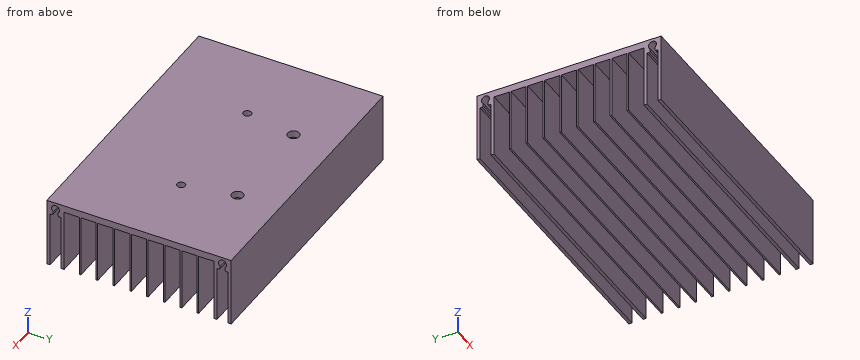
```python
from build123d import *

# Parameters (mm, degrees)
SCHIZZO1_W                   = 120
SCHIZZO1_H                   = 80
ESTRUSIONE_ESTRUSIONE1_DEPTH = 30
SCHIZZO2_W                   = 27
SCHIZZO2_H                   = 6.6
TAGLIO_ESTRUSIONE1_DEPTH     = 121
RIPETIZIONE_A_L1_COUNT       = 9
RIPETIZIONE_A_L1_PITCH       = 7.3
SCHIZZO3_W                   = 24
SCHIZZO3_H                   = 4.7
TAGLIO_ESTRUSIONE2_DEPTH     = 121
TAGLIO_ESTRUSIONE3_DEPTH     = 121
SMUSSO1_SIZE                 = 0.5
SCHIZZO5_R                   = 1.75
SCHIZZO5_R_2                 = 2.5
TAGLIO_ESTRUSIONE4_DEPTH     = 10


with BuildPart() as part:
    # Schizzo1 → Estrusione-Estrusione1 (new body)
    with BuildSketch(Plane.XY):
        Rectangle(SCHIZZO1_W, SCHIZZO1_H)
    extrude(amount=ESTRUSIONE_ESTRUSIONE1_DEPTH)

    # Schizzo2 → Taglio-Estrusione1 (cut, through all)
    with BuildSketch(Plane.ZY.offset(60)):
        with Locations((13.5, -29.2)):
            Rectangle(SCHIZZO2_W, SCHIZZO2_H)
    taglio_estrusione1 = extrude(amount=-TAGLIO_ESTRUSIONE1_DEPTH, mode=Mode.SUBTRACT)

    # Ripetizione a L1: Taglio-Estrusione1 ×9
    with Locations(*[(0, i * RIPETIZIONE_A_L1_PITCH, 0) for i in range(1, RIPETIZIONE_A_L1_COUNT)]):
        add(taglio_estrusione1, mode=Mode.SUBTRACT)

    # Schizzo3 → Taglio-Estrusione2 (cut, through all)
    with BuildSketch(Plane(origin=(60, 0, 0), x_dir=(0, 0, -1), z_dir=(1, 0, 0))):
        with Locations((-12, -36.25)):
            Rectangle(SCHIZZO3_W, SCHIZZO3_H)
        with Locations((-12, 36.25)):
            Rectangle(SCHIZZO3_W, SCHIZZO3_H)
    extrude(amount=-TAGLIO_ESTRUSIONE2_DEPTH, mode=Mode.SUBTRACT)

    # Schizzo4 → Taglio-Estrusione3 (cut, through all)
    with BuildSketch(Plane(origin=(60, 0, 0), x_dir=(0, 0, -1), z_dir=(1, 0, 0))):
        with BuildLine():
            ThreePointArc((-25.3, 36.25), (-25.38030749, 35.725951413), (-25.613859338, 35.25))
            Line((-25.613859338, 35.25), (-24, 35.25))
            Line((-24, 35.25), (-24, 37.25))
            Line((-24, 37.25), (-25.613859338, 37.25))
            ThreePointArc((-25.613859338, 37.25), (-25.38030749, 36.774048587), (-25.3, 36.25))
        make_face()
        with BuildLine():
            Line((-27.05, 37.25), (-27.05, 35.25))
            Line((-27.05, 35.25), (-25.613859338, 35.25))
            ThreePointArc((-25.613859338, 35.25), (-25.38030749, 35.725951413), (-25.3, 36.25))
            ThreePointArc((-25.3, 36.25), (-25.38030749, 36.774048587), (-25.613859338, 37.25))
            Line((-25.613859338, 37.25), (-27.05, 37.25))
        make_face()
        with BuildLine():
            Line((-25.613859338, 35.25), (-27.05, 35.25))
            Line((-27.05, 35.25), (-27.05, 37.25))
            Line((-27.05, 37.25), (-25.613859338, 37.25))
            ThreePointArc((-25.613859338, 37.25), (-28.8, 36.25), (-25.613859338, 35.25))
        make_face()
        with BuildLine():
            ThreePointArc((-25.3, -36.25), (-25.38030749, -35.725951413), (-25.613859338, -35.25))
            Line((-25.613859338, -35.25), (-27.05, -35.25))
            Line((-27.05, -35.25), (-27.05, -37.25))
            Line((-27.05, -37.25), (-25.613859338, -37.25))
            ThreePointArc((-25.613859338, -37.25), (-25.38030749, -36.774048587), (-25.3, -36.25))
        make_face()
        with BuildLine():
            Line((-27.05, -35.25), (-25.613859338, -35.25))
            ThreePointArc((-25.613859338, -35.25), (-28.8, -36.25), (-25.613859338, -37.25))
            Line((-25.613859338, -37.25), (-27.05, -37.25))
            Line((-27.05, -37.25), (-27.05, -35.25))
        make_face()
        with BuildLine():
            Line((-24, -37.25), (-24, -35.25))
            Line((-24, -35.25), (-25.613859338, -35.25))
            ThreePointArc((-25.613859338, -35.25), (-25.38030749, -35.725951413), (-25.3, -36.25))
            ThreePointArc((-25.3, -36.25), (-25.38030749, -36.774048587), (-25.613859338, -37.25))
            Line((-25.613859338, -37.25), (-24, -37.25))
        make_face()
    extrude(amount=-TAGLIO_ESTRUSIONE3_DEPTH, mode=Mode.SUBTRACT)

    # Smusso1
    smusso1_edges = [part.edges().sort_by_distance(p)[0] for p in [
        (0, 37.25, 24),
        (0, 35.25, 24),
        (0, -35.25, 24),
        (0, -37.25, 24),
    ]]
    chamfer(smusso1_edges, length=SMUSSO1_SIZE)

    # Schizzo5 → Taglio-Estrusione4 (cut)
    with BuildSketch(Plane.XY.offset(30)):
        with Locations((-25.5, 0)):
            Circle(SCHIZZO5_R)
        with Locations((26.686198964, 0)):
            Circle(SCHIZZO5_R)
        with Locations((-21.944553743, 22)):
            Circle(SCHIZZO5_R_2)
        with Locations((22.18196976, 22)):
            Circle(SCHIZZO5_R_2)
    extrude(amount=-TAGLIO_ESTRUSIONE4_DEPTH, mode=Mode.SUBTRACT)


solid = part.part
```
Here's how the part is built. I have some questions about the finished solid (model axes, mm). Coordinates: 2 decimals unless noted, no trailing zeros. Order: outer loops, then holes, each group sorted by start corner. A loop starts at its lowest first (then second) coordinate and runs counter-clockwise, first axis right, second up.
1) Imagine slicing it at C-C on y = 22. List the corners of the cut face in (x, z) for me.
2) Imagine slicing it at B-B on z = 11.25. State how many separate pieces and enclosed holes the cut face has, and give its area (3 significant figures).
3) Imagine slicing it at A-A on y = 0. List the corners of the cut face in (x, z) for me.
4) Imagine slicing it at D-D on y = -28. List the corners of the cut face in (x, z) for me.
5) I need wall thicknesses on line 1 (Y direction, x = -6.5, z = 27.05); line 2 (Z direction, x = -9.5, y = -21); line 3 (Y direction, x = -25.5, z = 28.6). Which ranges of each line are inside material? Lowest first, please.
6) Will this pin go through, and if not, where does the flat tip stop? pin 1 (6 mm diameter, centred on x = 23, y = 7.5, fed in from -Z).
Response values:
1. outline: (-60, 27) - (-24.44, 27) - (-24.44, 30) - (-60, 30) - close; (-19.44, 27) - (19.68, 27) - (19.68, 30) - (-19.44, 30) - close; (24.68, 27) - (60, 27) - (60, 30) - (24.68, 30) - close
2. separate pieces: 12
2. enclosed holes: 0
2. area: 1,340 mm2
3. outline: (-60, 27) - (-27.25, 27) - (-27.25, 30) - (-60, 30) - close; (-23.75, 27) - (24.94, 27) - (24.94, 30) - (-23.75, 30) - close; (28.44, 27) - (60, 27) - (60, 30) - (28.44, 30) - close
4. outline: (-60, 27) - (60, 27) - (60, 30) - (-60, 30) - close
5. line 1: y = -40 to -38, -34.5 to 34.5, 38 to 40
5. line 2: z = 27 to 30
5. line 3: y = -40 to -37.06, -35.44 to -1.75, 1.75 to 35.44, 37.06 to 40
6. pin 1: stops at z = 27
